Could you check a few things on this model? Use its own coordinates, in mm. A direction names the side the tool comes from. Coordinates: 2 decimals unless noted, no trailing zeros. Loops run counter-clockwise (first coordinate to the right, second up) from the corner with the lowest first, then second, coordinate; pieces in that order, holes last. Notation, with made-up numbers: (7.5, -39) - (66.5, -39) arc R21 cw to (66.5, 0) - close; hole circle Ø8 at (48.5, -5.5). An arc over 180 degrees is marked (long way). Put each result on its own line as item: value. Start each with the question number.
```python
from build123d import *

# Parameters (mm, degrees)
EXTRUDE_1_DEPTH     = 0.8
CUT_EXTRUDE_1_REACH = 2.8
SKETCH_2_R          = 1.25
EXTRUDE_2_DEPTH     = 5


with BuildPart() as part:
    # 草图1 → 凸台-拉伸1 (new body)
    with BuildSketch(Plane.XY):
        with BuildLine():
            Line((-4.76744186, 6.351378938), (3.23255814, 6.351378938))
            ThreePointArc((3.23255814, 6.351378938), (3.939664921, 6.058485719), (4.23255814, 5.351378938))
            Line((4.23255814, 5.351378938), (4.23255814, -5.648621062))
            ThreePointArc((4.23255814, -5.648621062), (3.939664921, -6.355727843), (3.23255814, -6.648621062))
            Line((3.23255814, -6.648621062), (-4.76744186, -6.648621062))
            ThreePointArc((-4.76744186, -6.648621062), (-5.474548642, -6.355727843), (-5.76744186, -5.648621062))
            Line((-5.76744186, -5.648621062), (-5.76744186, 5.351378938))
            ThreePointArc((-5.76744186, 5.351378938), (-5.474548642, 6.058485719), (-4.76744186, 6.351378938))
        make_face()
    extrude(amount=EXTRUDE_1_DEPTH)

    # 草图2 → 切除-拉伸1 (cut, up to next)
    with BuildSketch(Plane(origin=(0, 0, 0), x_dir=(-1, 0, 0), z_dir=(0, 0, -1)), mode=Mode.PRIVATE) as cut_extrude_1_sk1:
        with Locations((0.76744186, 3.751378938)):
            Circle(SKETCH_2_R)
    cut_extrude_1_tool1 = extrude(cut_extrude_1_sk1.sketch, amount=-CUT_EXTRUDE_1_REACH, mode=Mode.PRIVATE) & part.part
    add(cut_extrude_1_tool1.solids().sort_by_distance((-0.767442, 3.751379, 0))[0], mode=Mode.SUBTRACT)

    # 草图3 → 凸台-拉伸2 (add)
    with BuildSketch(Plane(origin=(0, 0, 0), x_dir=(-1, 0, 0), z_dir=(0, 0, -1))):
        with BuildLine():
            Line((-1.98255814, -4.648621062), (3.51744186, -4.648621062))
            ThreePointArc((3.51744186, -4.648621062), (4.26744186, -5.398621062), (3.51744186, -6.148621062))
            Line((3.51744186, -6.148621062), (-1.98255814, -6.148621062))
            ThreePointArc((-1.98255814, -6.148621062), (-2.73255814, -5.398621062), (-1.98255814, -4.648621062))
        make_face()
    extrude(amount=EXTRUDE_2_DEPTH)


solid = part.part
```
(1) I want a section at C-C on y = -4. List the corners of the cut face in (x, z) for me, and give its area (3 significant figures).
(2) If we mould it in two halves opening along Y, with no side actions, what happens to faces 1 (the cylindrical face through (-5.47, -6.36, 0.39)), 2 (the cylindrical face through (-5.482, 6.051, 0.394)), 3 (the cylindrical face through (2.732, -5.415, -2.465)), 4 (the cylindrical face through (-1.92, 3.27, 0.39))? For each: pulls with the +Y half, pulls with the -Y half, needs draft (parallel to the pull), parting line crosses it, or undercut.
(3) I want a section at A-A on x = -2.25. List the corners of the cut face in (y, z) for me, and give its area (3 significant figures).
(4) I want a section at B-B on x = -1. List the corners of the cut face in (y, z) for me.
(5) I need wall thicknesses on L1, parallel to Y at x = 0.5, z = -1.35; L2, parallel to Z at x = -3.5, y = 4.5; L3, parallel to Y at x = -4, z = -1.5. Which ranges of each line are inside material? Lowest first, please. Write a range as [from, to].
(6) For pin 1 Ø1.5 at (x, z) = (0, -3) entering from -Y; pin 2 Ø2 at (x, z) = (-4.5, -3) entering from +Y, each with a flat end and sliding along its axis, tell me the tip position at first contact or that it passes through.
(7) I want a section at D-D on z = -2.65. List the corners of the cut face in (x, y) for me, and give its area (3 significant figures).
(8) Which directions (+Z, -Z, +X, -X, +Y, -Y) give clear straight access to the entire face, cutting with the end or side of a thin tool? Please do faces 5 (the flat face through (-1, -6.149, -2)), 6 (the cylindrical face through (-4.267, -5.382, -2.465)), 7 (the flat face through (-1, -4.649, -2)), 8 (the cylindrical face through (3.93, 6.07, 0.39)), 9 (the flat face through (-1, 0, 0.8)).
Answer sheet:
1. outline: (-5.77, 0) - (4.23, 0) - (4.23, 0.8) - (-5.77, 0.8) - close
1. area: 8.00 mm^2
2. face 1: pulls with the -Y half
2. face 2: pulls with the +Y half
2. face 3: parting line crosses it
2. face 4: undercut
3. outline: (-6.65, 0) - (-6.15, 0) - (-6.15, -5) - (-4.65, -5) - (-4.65, 0) - (6.35, 0) - (6.35, 0.8) - (-6.65, 0.8) - close
3. area: 17.9 mm^2
4. outline: (-6.65, 0) - (-6.15, 0) - (-6.15, -5) - (-4.65, -5) - (-4.65, 0) - (2.52, 0) - (2.52, 0.8) - (-6.65, 0.8) - close; (4.98, 0) - (6.35, 0) - (6.35, 0.8) - (4.98, 0.8) - close
5. L1: y = [-6.15, -4.65]
5. L2: z = [0, 0.8]
5. L3: y = [-5.97, -4.82]
6. pin 1: stops at y = -6.15
6. pin 2: stops at y = -4.65
7. outline: (-3.52, -6.15) - (1.98, -6.15) arc R0.75 ccw to (1.98, -4.65) - (-3.52, -4.65) arc R0.75 ccw to start
7. area: 10.0 mm^2
8. face 5: -Z, +X, -X, -Y
8. face 6: -Z, -X
8. face 7: -Z, +X, -X, +Y
8. face 8: +Z, -Z, +X, +Y
8. face 9: +Z, +X, -X, +Y, -Y
